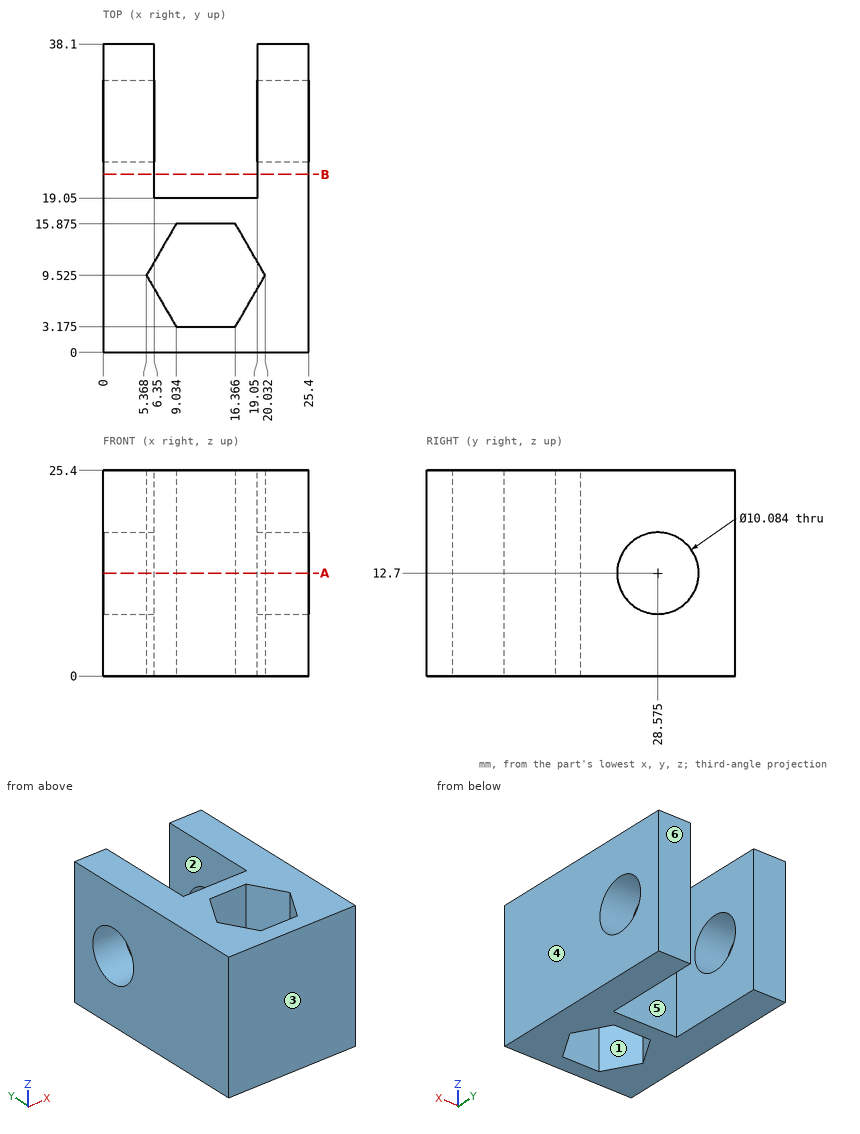
Here's the drawing with two shaded views (mm, measured from the low corner). I have some questions. A direction names the side the tool comes from. Give positions to 0.01 mm unless a question says otherwise; leave off trailing zeros. Write each loop counter-clockwise with the first axis right and the second up, starting at its lowest first coordinate (ties: lowest second). Pieces come first, ordered by that corner, then holes. Notation, with made-up numbers: (53, 67) -> (88, 67) arc R20 cw to (88, 82) -> close; hole circle Ø2 at (81.5, 45.25). An arc over 180 degrees is marked (long way). Use one line per item in the form item = value. Start each with the question number.
1. If I drill on L1, parallel to X at y = 35, z = 16.25; L2, parallel to Z at x = 19.5, y = 29.5, over which ranges is the centre line in solid material (lowest first)?
2. Will these pins go through, and if not, where does the flat tip stop? pin 1 Ø4 at (x, z) = (11, 11) entering from +Y; pin 2 Ø6 at (y, z) = (28.575, 12.7) entering from +X.
3. Imagine slicing it at A-A on z = 12.7. State how many separate pieces and enclosed holes the cut face has, plus the area to 3 significant figures.
4. On a 3-axis mill with a long thin cutter (end or side, diameter ignored), from which of +Z, -Z, +X, -X, +Y, -Y can I reach the whole of each face in a straight line? I mean the marked faces 1, 2 and 3. Say none if no direction works.
5. Thinking about a two-plate mould opening in X: for the marked faces 4, 5 and 6, which applies, +X half, -X half, draft (parallel to the pull), parting line (faces both ways), or undercut?
6. Imagine slicing it at B-B on y = 22. List the corners of the cut face in (x, z) for me.
Entries:
q1.L1 = 0 to 6.35, 19.05 to 25.4
q1.L2 = 0 to 7.74, 17.66 to 25.4
q2.pin_1 = 19.05
q2.pin_2 = through
q3.separate_pieces = 3
q3.enclosed_holes = 1
q3.area = 458 mm²
q4.face_1 = +Z, -Z
q4.face_2 = +Z, -Z, +Y
q4.face_3 = +Z, -Z, +X, -X, -Y
q5.face_4 = +X half
q5.face_5 = undercut
q5.face_6 = draft
q6.outline = (0, 0) -> (6.35, 0) -> (6.35, 25.4) -> (0, 25.4) -> close; (19.05, 0) -> (25.4, 0) -> (25.4, 25.4) -> (19.05, 25.4) -> close
